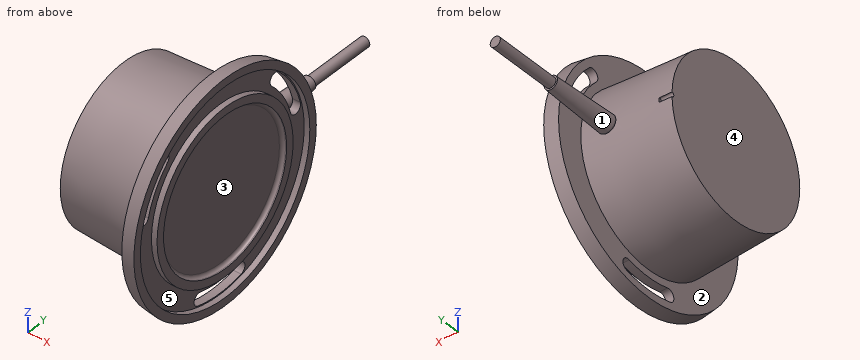
```python
from build123d import *

# Parameters (mm, degrees)
ESQUISSE2_R                  = 1
ENL_V_MAT_EXTRU_1_DEPTH      = 5.5
ESQUISSE3_R                  = 4
EXTRUSION1_DEPTH             = 36
ESQUISSE4_R                  = 4
EXTRUSION2_DEPTH             = 30
EXTRUSION2_TAPER             = 2
ESQUISSE5_R                  = 2.25
EXTRUSION3_DEPTH             = 30
ENL_V_MAT_EXTRU_2_DEPTH      = 7
R_P_TITION_CIRCULAIRE1_COUNT = 3


with BuildPart() as part:
    # Esquisse1 → Révolution1 (revolve)
    with BuildSketch(Plane.XY):
        with BuildLine():
            Line((0, 0), (0, 34.5))
            Line((0, 34.5), (39, 36.5))
            Line((39, 36.5), (39, 48.5))
            Line((39, 48.5), (45, 49.25))
            Line((45, 49.25), (45, 45.75))
            Line((45, 45.75), (42.5, 45.75))
            Line((42.5, 45.75), (42.5, 36.75))
            Line((42.5, 36.75), (45, 36.75))
            Line((45, 36.75), (45, 33.25))
            Line((45, 33.25), (44.5, 33.25))
            ThreePointArc((44.5, 33.25), (43.439339828, 32.810660172), (43, 31.75))
            Line((43, 31.75), (43, 0))
            Line((43, 0), (0, 0))
        make_face()
    revolve(axis=Axis((104.922362869, 0, 0), (-1, 0, 0)))

    # Esquisse2 → Enlèv. mat.-Extru.1 (cut)
    with BuildSketch(Plane.ZY):
        with Locations((0, 34.5)):
            Circle(ESQUISSE2_R)
    extrude(amount=-ENL_V_MAT_EXTRU_1_DEPTH, mode=Mode.SUBTRACT)

    # Esquisse3 → Extrusion1 (add)
    with BuildSketch(Plane(origin=(0, 0, 0), x_dir=(1, 0, 0), z_dir=(0, 1, 0))):
        with Locations((28, 0)):
            Circle(ESQUISSE3_R)
    extrude(amount=EXTRUSION1_DEPTH)

    # Esquisse4 → Extrusion2 (add)
    with BuildSketch(Plane(origin=(0, 36, 0), x_dir=(-1, 0, 0), z_dir=(0, 1, 0))):
        with Locations((-28, 0)):
            Circle(ESQUISSE4_R)
    extrude(amount=EXTRUSION2_DEPTH, taper=EXTRUSION2_TAPER)

    # Esquisse5 → Extrusion3 (add)
    with BuildSketch(Plane(origin=(0, 66, 0), x_dir=(-1, 0, 0), z_dir=(0, 1, 0))):
        with Locations((-28, 0)):
            Circle(ESQUISSE5_R)
    extrude(amount=EXTRUSION3_DEPTH)

    # Esquisse6 → Enlèv. mat.-Extru.2 (cut, through all)
    with BuildSketch(Plane.ZY.offset(-39)):
        with BuildLine():
            ThreePointArc((-38.395503832, 10.288235294), (-40.340031844, 13.656292718), (-43.708089268, 11.711764706))
            ThreePointArc((-43.708089268, 11.711764706), (-45.25, 0), (-43.708089268, -11.711764706))
            ThreePointArc((-43.708089268, -11.711764706), (-40.340031844, -13.656292718), (-38.395503832, -10.288235294))
            ThreePointArc((-38.395503832, -10.288235294), (-39.75, 0), (-38.395503832, 10.288235294))
        make_face()
    enl_v_mat_extru_2 = extrude(amount=-ENL_V_MAT_EXTRU_2_DEPTH, mode=Mode.SUBTRACT)

    # Répétition circulaire1: Enlèv. mat.-Extru.2 ×3 about axis
    r_p_tition_circulaire1_axis = Axis((39, 0, 0), (-1, 0, 0))
    for i in range(1, R_P_TITION_CIRCULAIRE1_COUNT):
        add(enl_v_mat_extru_2.rotate(r_p_tition_circulaire1_axis, i * 360 / R_P_TITION_CIRCULAIRE1_COUNT), mode=Mode.SUBTRACT)


solid = part.part
```
Verification items for the finished model (mm, model axes). Face numbers are marked on the shaded views. A direction names the side the tool comes from. Round coordinates to 2 decimals unless told otherwise and drop trailing zeros. Order: outer loops, then holes, each group sorted by start corner. A loop starts at its lowest first (then second) coordinate and runs counter-clockwise, first axis right, second up. Notation, with made-up numbers: (53, 74) - (65, 74) arc R7 ccw to (65, 84) - close; hole circle Ø8 at (60, 31.5). An arc over 180 degrees is marked (long way). Use CSV: the item, a comma, the result in double quotes.
(1) Gauge pin test, flat ends, axial feed: pin 1 Ø1 at (x, y) = (26.5, 74.5) entering from -Z; pin 2 Ø5 at (x, y) = (23.5, 15) entering from -Z; pin 3 Ø4 at (x, z) = (15.5, -23) entering from +Y. Record the tip position at first contact, or that the pin passes through.
Entries:
pin 1,"z = -2.02"
pin 2,"z = -33.46"
pin 3,"y = 28.37"
(2) Section check B-B on y = 82.5. Record the boundary of the cut face in (x, z).
Entries:
outline,"circle Ø4.5 at (28, 0)"
(3) Access from +Z, -Z, +X, -X, +Y, -Y to the whole of each face (thin tool, end or side, straight path). Record for the marked faces 4 and 5.
Entries:
face 4,"+Z, -Z, -X, +Y, -Y"
face 5,"+X"
(4) Thickness scan on probe 1 along Y at (x, z) = (44.9, 0); probe 2 along Z at (x, y) = (44.8, 0) (3 decimals); probe 3 along Y at (x, z) = (44, 0) (3 decimals). Record the ranges inside material, lowest first. Write a range as from..to.
Entries:
probe 1,"-49.24..-45.75, -36.75..-33.25, 33.25..36.75, 45.75..49.24"
probe 2,"-49.225..-45.75, -36.75..-33.25, 33.25..36.75, 45.75..49.225"
probe 3,"-49.125..-45.75, -36.75..-33.164, 33.164..36.75, 45.75..49.125"
(5) Section check C-C on x = 35.5. Record the boundary of the cut face in (y, z), and give its area (3 significant figures).
Entries:
outline,"circle Ø72.64 at (0, 0)"
area,"4,140 mm^2"
(6) Mould release check, pull along Y, two halves, no side actions. Record for the marked faces 1, 2 and 3: released by +Y, released by -Y, zero draft, split by the parting line, or undercut.
Entries:
face 1,"released by +Y"
face 2,"zero draft"
face 3,"undercut"
(7) Section check A-A on y = 0. Record the boundary of the cut face in (x, z).
Entries:
outline,"(0, -34.5) - (39, -36.5) - (39, -39.75) - (42.5, -39.75) - (42.5, -36.75) - (45, -36.75) - (45, -33.25) - (44.5, -33.25) arc R1.5 cw to (43, -31.75) - (43, 31.75) arc R1.5 cw to (44.5, 33.25) - (45, 33.25) - (45, 36.75) - (42.5, 36.75) - (42.5, 45.75) - (45, 45.75) - (45, 49.25) - (39, 48.5) - (39, 36.5) - (0, 34.5) - close; (39, -48.5) - (45, -49.25) - (45, -45.75) - (42.5, -45.75) - (42.5, -45.25) - (39, -45.25) - close"
